Geometry check sheet. Reference: the model listing, model coordinates, mm. A direction names the side the tool comes from. Give positions to 0.01 mm unless a question says otherwise; leave off trailing zeros. Loops run counter-clockwise (first coordinate to the right, second up) from the corner with the lowest first, then second, coordinate; pieces in that order, holes last. Notation, with made-up numbers: (88, -23) -> (141, -23) arc R21 cw to (141, 13) -> close; hole circle Ø8 at (64, 76.25). An arc over 180 degrees is marked (long way). One line per question, with ' | ' between items.
from build123d import *

# Parameters (mm, degrees)
SKIZZE4_W                       = 50
SKIZZE4_H                       = 50
AUFSATZ_LINEAR_AUSTRAGEN1_DEPTH = 150
SKIZZE5_W                       = 50
SKIZZE5_H                       = 50
AUFSATZ_LINEAR_AUSTRAGEN2_DEPTH = 25
SKIZZE6_R                       = 5
SCHNITT_LINEAR_AUSTRAGEN1_DEPTH = 75
SKIZZE8_R                       = 5
SCHNITT_LINEAR_AUSTRAGEN2_DEPTH = 50
SCHNITT_LINEAR_AUSTRAGEN3_DEPTH = 75
SCHNITT_LINEAR_AUSTRAGEN4_DEPTH = 25
SKIZZE11_R                      = 21.1
SKIZZE11_R_2                    = 12.4
SCHNITT_LINEAR_AUSTRAGEN5_DEPTH = 5
SKIZZE12_R                      = 10.2
SKIZZE12_R_2                    = 10
SCHNITT_LINEAR_AUSTRAGEN6_DEPTH = 5.5
SKIZZE13_R                      = 10
SCHNITT_LINEAR_AUSTRAGEN7_DEPTH = 6
SCHNITT_LINEAR_START            = -5.5
SKIZZE14_R                      = 10
SCHNITT_LINEAR_AUSTRAGEN8_DEPTH = 5.5


with BuildPart() as part:
    # Skizze4 → Aufsatz-Linear austragen1 (new body)
    with BuildSketch(Plane(origin=(0, 0, 0), x_dir=(1, 0, 0), z_dir=(0, 1, 0))):
        Rectangle(SKIZZE4_W, SKIZZE4_H)
    extrude(amount=AUFSATZ_LINEAR_AUSTRAGEN1_DEPTH)

    # Skizze5 → Aufsatz-Linear austragen2 (add)
    with BuildSketch(Plane.XY.offset(25)):
        with Locations((0, 125)):
            Rectangle(SKIZZE5_W, SKIZZE5_H)
    extrude(amount=AUFSATZ_LINEAR_AUSTRAGEN2_DEPTH)

    # Skizze6 → Schnitt-Linear austragen1 (cut)
    with BuildSketch(Plane.XY.offset(50)):
        with Locations((0, 125)):
            Circle(SKIZZE6_R)
    extrude(amount=-SCHNITT_LINEAR_AUSTRAGEN1_DEPTH, mode=Mode.SUBTRACT)

    # Skizze8 → Schnitt-Linear austragen2 (cut)
    with BuildSketch(Plane.XY.offset(25)):
        with BuildLine():
            ThreePointArc((0, 0), (-17.67766953, 7.32233047), (-25, 25))
            Line((-25, 25), (-25, 0))
            Line((-25, 0), (0, 0))
        make_face()
        with BuildLine():
            ThreePointArc((25, 25), (17.67766953, 7.32233047), (0, 0))
            Line((0, 0), (25, 0))
            Line((25, 0), (25, 25))
        make_face()
        with Locations((0, 25)):
            Circle(SKIZZE8_R)
    extrude(amount=-SCHNITT_LINEAR_AUSTRAGEN2_DEPTH, mode=Mode.SUBTRACT)

    # Skizze9 → Schnitt-Linear austragen3 (cut)
    with BuildSketch(Plane.XY.offset(50)):
        with BuildLine():
            Line((0, 150), (-25, 150))
            Line((-25, 150), (-25, 125))
            ThreePointArc((-25, 125), (-17.67766953, 142.67766953), (0, 150))
        make_face()
        with BuildLine():
            Line((25, 150), (0, 150))
            ThreePointArc((0, 150), (17.67766953, 142.67766953), (25, 125))
            Line((25, 125), (25, 150))
        make_face()
    extrude(amount=-SCHNITT_LINEAR_AUSTRAGEN3_DEPTH, mode=Mode.SUBTRACT)

    # Skizze10 → Schnitt-Linear austragen4 (cut)
    with BuildSketch(Plane.XY.offset(50)):
        with BuildLine():
            ThreePointArc((0, 100), (-17.67766953, 107.32233047), (-25, 125))
            Line((-25, 125), (-25, 100))
            Line((-25, 100), (0, 100))
        make_face()
        with BuildLine():
            Line((25, 100), (25, 125))
            ThreePointArc((25, 125), (17.67766953, 107.32233047), (0, 100))
            Line((0, 100), (25, 100))
        make_face()
    extrude(amount=-SCHNITT_LINEAR_AUSTRAGEN4_DEPTH, mode=Mode.SUBTRACT)

    # Skizze11 → Schnitt-Linear austragen5 (cut)
    with BuildSketch(Plane.XY.offset(50)):
        with Locations((0, 125)):
            Circle(SKIZZE11_R)
        with Locations((0, 125)):
            Circle(SKIZZE11_R_2, mode=Mode.SUBTRACT)
    extrude(amount=-SCHNITT_LINEAR_AUSTRAGEN5_DEPTH, mode=Mode.SUBTRACT)

    # Skizze12 → Schnitt-Linear austragen6 (cut)
    with BuildSketch(Plane(origin=(0, 0, -25), x_dir=(-1, 0, 0), z_dir=(0, 0, -1))):
        with Locations((0, 125)):
            Circle(SKIZZE12_R)
        with Locations((0, 25)):
            Circle(SKIZZE12_R_2)
    extrude(amount=-SCHNITT_LINEAR_AUSTRAGEN6_DEPTH, mode=Mode.SUBTRACT)

    # Skizze13 → Schnitt-Linear austragen7 (cut)
    with BuildSketch(Plane.XY.offset(50)):
        with Locations((0, 125)):
            Circle(SKIZZE13_R)
    extrude(amount=-SCHNITT_LINEAR_AUSTRAGEN7_DEPTH, mode=Mode.SUBTRACT)

    # Skizze14 → Schnitt-Linear austragen8 (cut)
    with BuildSketch(Plane.XY.offset(25).offset(SCHNITT_LINEAR_START)):
        with Locations(Location((0, 25, 0), (0, 0, 180))):
            Circle(SKIZZE14_R)
    extrude(amount=SCHNITT_LINEAR_AUSTRAGEN8_DEPTH, mode=Mode.SUBTRACT)


solid = part.part
Item 1: Sectioned sample at D-D (x = -2). Give the number of separate pieces and of enclosed holes in the cut face, plus the area to 3 significant figures.
Result:
separate pieces: 3 | enclosed holes: 0 | area: 7,270 mm2
Item 2: Release check for a two-part mould opening along Y. For faces 4 (the face through (-1.614, 137.294, 47.535)), 5 (the face through (-17, 112, 50)) record: pulls with the +Y half, pulls with the -Y half, needs draft (parallel to the pull), parting line crosses it, or undercut.
Result:
face 4: undercut | face 5: needs draft
Item 3: Sectioned sample at B-B (z = 40). Record the cut outline in (x, y), plus the area to 3 significant figures.
Result:
outline: circle Ø50 at (0, 125); hole circle Ø10 at (0, 125) | area: 1,880 mm2
Item 4: Set-up check for faces 1 (the face through (-0.651, 129.957, 12.694)), 2 (the face through (9, 116, 45)), 3 (the face through (-2, 130, -19.5)): record each of +Z, -Z, +X, -X, +Y, -Y from which the full face is reachable in a straight line by a thin tool's end or side.
Result:
face 1: +Z, -Z | face 2: +Z | face 3: -Z
Item 5: Scan lines: probe 1 along X at (y, z) = (25, 21); probe 2 along Y at (x, z) = (-1, 24); probe 3 along Z at (x, y) = (23, 95). Record each from-to range of solid material in increasing order.
Result:
probe 1: -25 to -10, 10 to 25 | probe 2: 0.02 to 15.05, 34.95 to 120.1, 129.9 to 149.98 | probe 3: -25 to 25
Item 6: Sectioned sample at A-A (z = 18). Record the cut outline in (x, y), plus the area to 3 significant figures.
Result:
outline: (-25, 25) arc R25 ccw to (25, 25) -> (25, 125) arc R25 ccw to (-25, 125) -> close; hole circle Ø10 at (0, 25); hole circle Ø10 at (0, 125) | area: 6,810 mm2
Item 7: Sectioned sample at C-C (y = 31.5). Record the cut outline in (x, z).
Result:
outline: (-25, -25) -> (-7.6, -25) -> (-7.6, -19.5) -> (7.6, -19.5) -> (7.6, -25) -> (25, -25) -> (25, 25) -> (7.6, 25) -> (7.6, 19.5) -> (-7.6, 19.5) -> (-7.6, 25) -> (-25, 25) -> close
Item 8: Depth check by flat-ended pin: pin 1 Ø16 at (x, y) = (0, 125) entering from -Z; pin 2 Ø15 at (x, y) = (-2.5, 62.5) entering from +Z; pin 3 Ø16 at (x, y) = (1.5, 125) entering from +Z. Enter the tip coordinate at first touch or a pass-through.
Result:
pin 1: z = -19.5 | pin 2: z = 25 | pin 3: z = 44
